Design review of the part built by this model. Coordinates are the model's own, in mm. A direction names the side the tool comes from. Give positions to 0.01 mm unless a question says otherwise; leave off trailing zeros. Loops run counter-clockwise (first coordinate to the right, second up) from the corner with the lowest first, then second, coordinate; pieces in that order, holes last. Notation, with made-up numbers: M 58.5,26 L 73.5,26 A24 cw 73.5,45 Z; hole C -37.5,84.25 d9. An arc over 180 degrees is marked long. Use CSV: the item, a comma, the result in double quotes.
from build123d import *

# Parameters (mm, degrees)
F1_DEPTH = 25


with BuildPart() as f1:
    # F0 (on Right) → F1 (new body)
    with BuildSketch(Plane.YZ):
        Polygon((-76.896277, 150.686045), (-76.896277, -349.313955), (-51.896277, -349.313955), (-51.896277, -49.313955), (-51.896277, -9.338717), (-51.896277, 94.751239), (19.953003, 94.751239), (57.223622, 94.751239), (223.103723, 94.751239), (223.103723, 150.690981), align=None)
        Polygon((-51.896277, -9.338717), (-51.896277, -49.313955), (57.223622, 94.751239), (19.953003, 94.751239), align=None)
    extrude(amount=F1_DEPTH)


solid = f1.part
(1) Wall thickness on line 1 along Y through (x, z) = (1.5, -208.5); line 2 along Z through (x, y) = (9.25, 125.5); line 3 along Z through (x, y) = (16.25, 13.5): over which ranges is each line inside the solid? List them lowest first. Write a range as [from, to].
A:
line 1,"[-76.9, -51.9]"
line 2,"[94.75, 150.69]"
line 3,"[37.03, 85.4], [94.75, 150.69]"
(2) We need section A-A on y = 10. State the section outline as (x, z) points.
A:
outline,"M 0,32.4 L 25,32.4 L 25,80.33 L 0,80.33 Z; M 0,94.75 L 25,94.75 L 25,150.69 L 0,150.69 Z"
(3) We need section C-C on x = 18. State the section outline as (y, z) points.
A:
outline,"M -76.9,-349.31 L -51.9,-349.31 L -51.9,-49.31 L 57.22,94.75 L 223.1,94.75 L 223.1,150.69 L -76.9,150.69 Z; hole M -51.9,-9.34 L 19.95,94.75 L -51.9,94.75 Z"
(4) We need section D-D on z = -282.5. State the section outline as (x, y) points, then the cut area to 3 significant figures.
A:
outline,"M 0,-76.9 L 25,-76.9 L 25,-51.9 L 0,-51.9 Z"
area,"625 mm²"
(5) Clearance check with flat-ended pins moving along their axes: P1, Ø7.5, axis at x = 10, z = -149, coming from the +Y side; P2, Ø7.5, axis at x = 10.5, y = -16.5, coming from the -Z side; P3, Ø6, axis at x = 7.5, y = -31.5, coming from the +Z side. State where each tip first meets the part, or that it passes through.
A:
P1,"y = -51.9"
P2,"z = -7.53"
P3,"z = 150.69"
(6) Machinability: for faces 4 (the flat face through (12, -51.896, -201)), 5 (the flat face through (12, -65, -349.314)), 6 (the flat face through (12, -51.896, 42)), which of the approach directions +Z, -Z, +X, -X, +Y, -Y give a long, thin tool a straight path to every point of the face, cutting with its end or side? Answer none if there is none.
A:
face 4,"-Z, +X, -X, +Y"
face 5,"-Z, +X, -X, +Y, -Y"
face 6,"+X, -X"
(7) We need section B-B on z = 25.5. State the section outline as (x, y) points, then the cut area to 3 significant figures.
A:
outline,"M 0,-76.9 L 25,-76.9 L 25,-51.9 L 0,-51.9 Z; M 0,-27.85 L 25,-27.85 L 25,4.77 L 0,4.77 Z"
area,"1,440 mm²"
(8) The part is to be moulded in two halves that separate along Z. For faces 1 (the flat face through (12, 139, 94.751)), 2 (the flat face through (12, -16, 94.751)), 3 (the flat face through (12, 223.104, 122)), say which applies: released by +Z, released by -Z, zero draft, split by the parting line, or undercut.
A:
face 1,"released by -Z"
face 2,"undercut"
face 3,"zero draft"
